Geometry check sheet. Reference: the model listing, model coordinates, mm. A direction names the side the tool comes from. Round coordinates to 2 decimals unless told otherwise and drop trailing zeros. Write each loop counter-clockwise with the first axis right and the second up, starting at its lowest first coordinate (ties: lowest second). Pieces come first, ordered by that corner, then holes.
Item 1: Cross-section at A-A (x = 4.7). Enter the section's corners in (y, z).
Item 2: Draft check along Z on faces 1 (the face through (31.66, 3.57, 5.14)), 2 (the face through (20.051, 0.789, 4.785)), 3 (the face through (30.465, 0.789, 8.199)), 4 (the face through (49.9, 0.81, 0.57)). Enter one of: pulls with the +Z half, pulls with the -Z half, needs draft (parallel to the pull), parting line crosses it, or undercut.
Item 3: Cross-section at B-B (x = 21.5). Enter the section's corners in (y, z), then the cut area to 3 significant figures.
Item 4: Cross-section at C-C (x = 32.75). Enter the section's corners in (y, z), then the cut area to 3 significant figures.
Item 5: Access from +Z, -Z, +X, -X, +Y, -Y to the whole of each face (thin tool, end or side, straight path). Record for faces 5 (the face through (6, 1, 6.5)), 6 (the face through (37.75, 1, 15)), 7 (the face through (15.551, 0.789, 21.715)).
Item 6: Cross-section at D-D (y = 4.55). Enter the section's corners in (x, z), then the cut area to 3 significant figures.
Item 7: Scan lines: probe 1 along X at (y, z) = (0.75, 3.7); probe 2 along Z at (x, y) = (45.8, 0.45); probe 3 along Y at (x, z) = (36, 3.25). Record each from-to range of solid material in increasing order.
Item 8: Depth check by flat-ended pin: P1, Ø0.8, axis at y = 1, z = 20.5, coming from the -X side; P2, Ø3, axis at x = 22.5, z = 19, coming from the +Y side; P3, Ø1.7, axis at x = 45.8, z = 3.7, coming from the +Y side; P4, Ø0.8, axis at x = 42, y = 0.5, coming from the +Z side. Enter the tip coordinate at first touch or a pass-through.
from build123d import *

# Parameters (mm, degrees)
SKIZZE1_R                       = 1.45
AUFSATZ_LINEAR_AUSTRAGEN1_DEPTH = 1.6
VERRUNDUNG1_R                   = 2
SKIZZE2_R                       = 1.1
AUFSATZ_LINEAR_AUSTRAGEN2_DEPTH = 4
SKIZZE3_W                       = 11
SKIZZE3_H                       = 4
SCHNITT_LINEAR_AUSTRAGEN1_DEPTH = 3
VERRUNDUNG2_R                   = 1
SKIZZE4_W                       = 20
SKIZZE4_H                       = 3
SCHNITT_LINEAR_AUSTRAGEN2_DEPTH = 3
VERRUNDUNG3_R                   = 1


with BuildPart() as part:
    # Skizze1 → Aufsatz-Linear austragen1 (new body)
    with BuildSketch(Plane(origin=(0, 0, 0), x_dir=(1, 0, 0), z_dir=(0, 1, 0))):
        Polygon((0, 0), (50.5, 0), (50.5, -6.5), (37.75, -6.5), (37.75, -23), (12.75, -23), (12.75, -6.5), (0, -6.5), align=None)
        with Locations(Location((4.7, -3.7, 0), (0, 0, 270))):
            Circle(SKIZZE1_R, mode=Mode.SUBTRACT)
        with Locations(Location((45.8, -3.7, 0), (0, 0, 90))):
            Circle(SKIZZE1_R, mode=Mode.SUBTRACT)
    extrude(amount=AUFSATZ_LINEAR_AUSTRAGEN1_DEPTH)

    # Verrundung1
    verrundung1_edges = [part.edges().sort_by_distance(p)[0] for p in [
        (0, 0.8, 0),
        (50.5, 0.8, 0),
        (50.5, 0.8, 6.5),
        (37.75, 0.8, 6.5),
        (37.75, 0.8, 23),
        (12.75, 0.8, 23),
        (12.75, 0.8, 6.5),
        (0, 0.8, 6.5),
    ]]
    fillet(verrundung1_edges, radius=VERRUNDUNG1_R)

    # Skizze2 → Aufsatz-Linear austragen2 (add)
    with BuildSketch(Plane(origin=(0, 1.6, 0), x_dir=(1, 0, 0), z_dir=(0, 1, 0))):
        with Locations(Location((17.75, -5, 0), (0, 0, 270))):
            Circle(SKIZZE2_R)
        with Locations(Location((32.75, -5, 0), (0, 0, 90))):
            Circle(SKIZZE2_R)
    extrude(amount=AUFSATZ_LINEAR_AUSTRAGEN2_DEPTH)

    # Skizze3 → Schnitt-Linear austragen1 (cut)
    with BuildSketch(Plane(origin=(0, 1.6, 0), x_dir=(1, 0, 0), z_dir=(0, 1, 0))):
        with Locations((25.25, -6.5)):
            Rectangle(SKIZZE3_W, SKIZZE3_H)
    extrude(amount=-SCHNITT_LINEAR_AUSTRAGEN1_DEPTH, mode=Mode.SUBTRACT)

    # Verrundung2
    verrundung2_edges = [part.edges().sort_by_distance(p)[0] for p in [
        (19.75, 0.8, 8.5),
        (19.75, 0.8, 4.5),
        (30.75, 0.8, 4.5),
        (30.75, 0.8, 8.5),
    ]]
    fillet(verrundung2_edges, radius=VERRUNDUNG2_R)

    # Skizze4 → Schnitt-Linear austragen2 (cut)
    with BuildSketch(Plane(origin=(0, 1.6, 0), x_dir=(1, 0, 0), z_dir=(0, 1, 0))):
        with Locations((25.25, -20.5)):
            Rectangle(SKIZZE4_W, SKIZZE4_H)
    extrude(amount=-SCHNITT_LINEAR_AUSTRAGEN2_DEPTH, mode=Mode.SUBTRACT)

    # Verrundung3
    verrundung3_edges = [part.edges().sort_by_distance(p)[0] for p in [
        (15.25, 0.8, 22),
        (15.25, 0.8, 19),
        (35.25, 0.8, 19),
        (35.25, 0.8, 22),
    ]]
    fillet(verrundung3_edges, radius=VERRUNDUNG3_R)


solid = part.part
Resolved:
1. outline: (0, 0) - (1.6, 0) - (1.6, 2.25) - (0, 2.25) - close; (0, 5.15) - (1.6, 5.15) - (1.6, 6.5) - (0, 6.5) - close
2. face 1: parting line crosses it
2. face 2: undercut
2. face 3: undercut
2. face 4: pulls with the -Z half
3. outline: (0, 0) - (1.6, 0) - (1.6, 4.5) - (0, 4.5) - close; (0, 8.5) - (1.6, 8.5) - (1.6, 19) - (0, 19) - close; (0, 22) - (1.6, 22) - (1.6, 23) - (0, 23) - close
3. area: 25.6 mm2
4. outline: (0, 0) - (1.6, 0) - (1.6, 3.9) - (5.6, 3.9) - (5.6, 6.1) - (1.6, 6.1) - (1.6, 19) - (0, 19) - close; (0, 22) - (1.6, 22) - (1.6, 23) - (0, 23) - close
4. area: 40.8 mm2
5. face 5: +Z, -X, +Y, -Y
5. face 6: +Z, +X, +Y, -Y
5. face 7: +Y, -Y
6. outline: circle Ø2.2 at (17.75, 5); circle Ø2.2 at (32.75, 5)
6. area: 7.60 mm2
7. probe 1: x = 0 to 3.25, 6.15 to 44.35, 47.25 to 50.5
7. probe 2: z = 0 to 2.25, 5.15 to 6.5
7. probe 3: y = 0 to 1.6
8. P1: stops at x = 12.75
8. P2: stops at y = 1.6
8. P3: passes through
8. P4: stops at z = 6.5
